Geometry check sheet. Reference: the model listing, model coordinates, mm. A direction names the side the tool comes from. Give positions to 0.01 mm unless a question says otherwise; leave off trailing zeros. Order: outer loops, then holes, each group sorted by start corner. A loop starts at its lowest first (then second) coordinate and runs counter-clockwise, first axis right, second up.
from build123d import *

# Parameters (mm, degrees)
F0_W     = 20
F0_H     = 20
F0_W_2   = 710
F0_H_2   = 260
F1_DEPTH = 300


with BuildPart() as f1:
    # F0 (on Front) → F1 (new body)
    with BuildSketch(Plane.XZ):
        with Locations((-39.431209, 10)):
            Rectangle(F0_W, F0_H)
        with Locations((325.568791, 10)):
            Rectangle(F0_W_2, F0_H)
        Polygon((-49.431209, 580), (-49.431209, 20), (-29.431209, 20), (-29.431209, 300), (-29.431209, 320), (-29.431209, 440), (-29.431209, 460), (-29.431209, 580), align=None)
        with Locations((690.568791, 10)):
            Rectangle(F0_W, F0_H)
        with Locations((-39.431209, 590)):
            Rectangle(F0_W, F0_H)
        Polygon((680.568791, 300), (680.568791, 20), (700.568791, 20), (700.568791, 300), (1330.568791, 300), (1330.568791, 320), (700.568791, 320), (680.568791, 320), align=None)
        Polygon((-29.431209, 600), (-29.431209, 580), (680.568791, 580), (700.568791, 580), (1330.568791, 580), (1330.568791, 600), align=None)
        with Locations((1340.568791, 590)):
            Rectangle(F0_W, F0_H)
        with Locations((1340.568791, 310)):
            Rectangle(F0_W, F0_H)
        with Locations((1340.568791, 450)):
            Rectangle(F0_W, F0_H_2)
        with Locations((325.568791, 450)):
            Rectangle(F0_W_2, F0_H)
        Polygon((700.568791, 580), (680.568791, 580), (680.568791, 460), (680.568791, 440), (680.568791, 320), (700.568791, 320), align=None)
        with Locations((325.568791, 310)):
            Rectangle(F0_W_2, F0_H)
    extrude(amount=F1_DEPTH)


solid = f1.part
Item 1: Sectioned sample at D-D (z = 530). Enter the section's corners in (x, y), and give its area (3 significant figures).
Reported:
outline: (-49.43, -300) - (-29.43, -300) - (-29.43, 0) - (-49.43, 0) - close; (680.57, -300) - (700.57, -300) - (700.57, 0) - (680.57, 0) - close; (1330.57, -300) - (1350.57, -300) - (1350.57, 0) - (1330.57, 0) - close
area: 18,000 mm2
Item 2: Gauge pin test, flat end, axial feed: pin 1 (5 mm diameter, centred on y = -249, z = 183, fed in from +X). Record the tip position at first contact, or that the pin passes through.
Reported:
pin 1: stops at x = 700.57
Item 3: Sectioned sample at C-C (y = -186). Enter the section's corners in (x, z), and give its area (3 significant figures).
Reported:
outline: (-49.43, 0) - (700.57, 0) - (700.57, 300) - (1350.57, 300) - (1350.57, 600) - (-49.43, 600) - close; hole (-29.43, 20) - (680.57, 20) - (680.57, 300) - (-29.43, 300) - close; hole (-29.43, 320) - (680.57, 320) - (680.57, 440) - (-29.43, 440) - close; hole (-29.43, 460) - (680.57, 460) - (680.57, 580) - (-29.43, 580) - close; hole (700.57, 320) - (1330.57, 320) - (1330.57, 580) - (700.57, 580) - close
area: 112,000 mm2
Item 4: Draft check along Z on faces 4 (the flat face through (544, 0, 301)), 5 (the flat face through (320, -148, 0)), 6 (the flat face through (321, -148, 300)), 7 (the flat face through (1330.569, -148, 448)). Enter one of: released by +Z, released by -Z, zero draft, split by the parting line, or undercut.
Reported:
face 4: zero draft
face 5: released by -Z
face 6: undercut
face 7: undercut
Item 5: Set-up check for faces 1 (the flat face through (700.569, -148, 148)), 2 (the flat face through (-29.431, -148, 158)), 3 (the flat face through (1350.569, -148, 448)): record each of +Z, -Z, +X, -X, +Y, -Y from which the full face is reachable in a straight line by a thin tool's end or side.
Reported:
face 1: -Z, +X, +Y, -Y
face 2: +Y, -Y
face 3: +Z, -Z, +X, +Y, -Y
Item 6: Sectioned sample at B-B (z = 52.5). Enter the section's corners in (x, y), and give its area (3 significant figures).
Reported:
outline: (-49.43, -300) - (-29.43, -300) - (-29.43, 0) - (-49.43, 0) - close; (680.57, -300) - (700.57, -300) - (700.57, 0) - (680.57, 0) - close
area: 12,000 mm2
Item 7: Scan lines: L1, parallel to Z at x = 46, y = -73; L2, parallel to X at y = -284, z = 488; L3, parallel to Z at x = 1064, y = -277.5. Record each from-to range of solid material in increasing order.
Reported:
L1: z = 0 to 20, 300 to 320, 440 to 460, 580 to 600
L2: x = -49.43 to -29.43, 680.57 to 700.57, 1330.57 to 1350.57
L3: z = 300 to 320, 580 to 600
Item 8: Sectioned sample at A-A (x = 1110.5). Enter the section's corners in (y, z).
Reported:
outline: (-300, 300) - (0, 300) - (0, 320) - (-300, 320) - close; (-300, 580) - (0, 580) - (0, 600) - (-300, 600) - close
